```python
from build123d import *

# Parameters (mm, degrees)
CORTE_EXTRUS_O1_DEPTH      = 1
CORTE_EXTRUS_O1_DEPTH_BACK = 51
RESSALTO_EXTRUS_O1_START   = -2
ESBO_O3_R                  = 1.6
RESSALTO_EXTRUS_O1_DEPTH   = 3
ESBO_O4_W                  = 67.372166219
ESBO_O4_H                  = 55.074072385
ESBO_O4_W_2                = 51.598524128
ESBO_O4_H_2                = 14
CORTE_EXTRUS_O2_DEPTH      = 6
CORTE_EXTRUS_O2_DEPTH_BACK = 16.5


with BuildPart() as part:
    # Esboço1 → Revolução1 (revolve)
    with BuildSketch(Plane.XY):
        Polygon((15, 37), (15.5, 37), (15.5, 13), (15, 13), (15, 10), (15.5, 10), (15.5, 0), (12.5, 0), (12.5, 50), (15.5, 50), (15.5, 40), (15, 40), align=None)
    revolve(axis=Axis((0, 0, 0), (0, 1, 0)))

    # Esboço2 → Corte-extrusão1 (cut, two sides)
    with BuildSketch(Plane(origin=(0, 50, 0), x_dir=(1, 0, 0), z_dir=(0, 1, 0))) as corte_extrus_o1_sk:
        with BuildLine():
            Line((-11.456439237, -5), (-14.671400751, -5))
            ThreePointArc((-14.671400751, -5), (0, -15.5), (14.671400751, -5))
            Line((14.671400751, -5), (11.456439237, -5))
            ThreePointArc((11.456439237, -5), (0, -12.5), (-11.456439237, -5))
        make_face()
    extrude(amount=CORTE_EXTRUS_O1_DEPTH, mode=Mode.SUBTRACT)
    extrude(corte_extrus_o1_sk.sketch, amount=-CORTE_EXTRUS_O1_DEPTH_BACK, mode=Mode.SUBTRACT)

    # Esboço3 → Ressalto-extrusão1 (add)
    with BuildSketch(Plane.XY.offset(RESSALTO_EXTRUS_O1_START)):
        with BuildLine():
            Line((-13.5, 49), (-20, 49))
            ThreePointArc((-20, 49), (-24, 45), (-20, 41))
            Line((-20, 41), (-13.5, 41))
            Line((-13.5, 41), (-13.5, 49))
        make_face()
        with Locations((-20, 45)):
            Circle(ESBO_O3_R, mode=Mode.SUBTRACT)
        with BuildLine():
            Line((13.5, 41), (13.5, 49))
            Line((13.5, 49), (20, 49))
            ThreePointArc((20, 49), (24, 45), (20, 41))
            Line((20, 41), (13.5, 41))
        make_face()
        with Locations((20, 45)):
            Circle(ESBO_O3_R, mode=Mode.SUBTRACT)
        with BuildLine():
            Line((13.5, 1), (20, 1))
            ThreePointArc((20, 1), (24, 5), (20, 9))
            Line((20, 9), (13.5, 9))
            Line((13.5, 9), (13.5, 1))
        make_face()
        with Locations((20, 5)):
            Circle(ESBO_O3_R, mode=Mode.SUBTRACT)
        with BuildLine():
            Line((-13.5, 9), (-13.5, 1))
            Line((-13.5, 1), (-20, 1))
            ThreePointArc((-20, 1), (-24, 5), (-20, 9))
            Line((-20, 9), (-13.5, 9))
        make_face()
        with Locations((-20, 5)):
            Circle(ESBO_O3_R, mode=Mode.SUBTRACT)
    extrude(amount=-RESSALTO_EXTRUS_O1_DEPTH)

    # Esboço4 → Corte-extrusão2 (cut, two sides)
    with BuildSketch(Plane.XY) as corte_extrus_o2_sk:
        with Locations((0.066837467, 24.799487601)):
            Rectangle(ESBO_O4_W, ESBO_O4_H)
        with Locations((0, 42)):
            Rectangle(ESBO_O4_W_2, ESBO_O4_H_2, mode=Mode.SUBTRACT)
    extrude(amount=CORTE_EXTRUS_O2_DEPTH, mode=Mode.SUBTRACT)
    extrude(corte_extrus_o2_sk.sketch, amount=-CORTE_EXTRUS_O2_DEPTH_BACK, mode=Mode.SUBTRACT)


solid = part.part
```
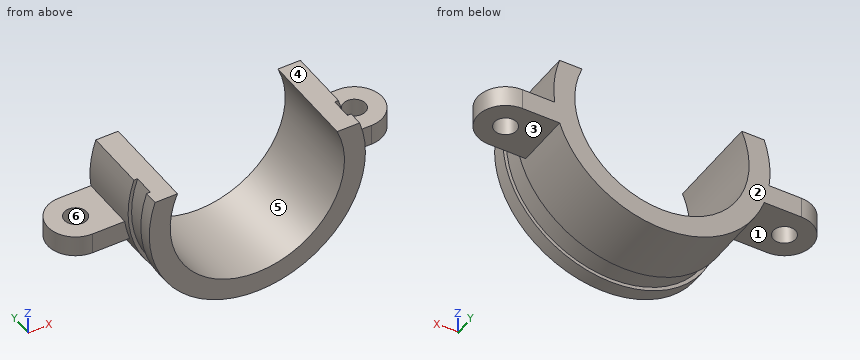
The listing builds one solid part. Answer for the finished solid, in the listing's coordinates (mm). Face numbers are marked on the shaded views. A direction names the side the tool comes from. Give positions to 0.01 mm unless a question says otherwise; leave off trailing zeros. Write each loop counter-clockwise with the first axis right and the second up, starting at its lowest first coordinate (ties: lowest second). Pieces come first, ordered by that corner, then holes. Notation, with made-up numbers: M -19.75,-32 L 18.25,-32 A23 cw 18.25,-8 Z; hole C 44.25,75 d4. An arc over 180 degrees is marked long. Write each question's results on one line, items separated by ' | '.
Q1. Consider L1, parallel to Y at x = -20, z = -4.4; L2, parallel to X at y = 43.75, z = 0; L3, parallel to Y at x = 6, z = -14. Determine where each line is inside the solid, lowest interval first. Write a range as from..to.
Output values:
L1: 41..43.4, 46.6..49 | L2: -15.5..-12.5, 12.5..15.5 | L3: 35..37, 40..49
Q2. Section C-C, the plane x = 0 is taken. Write down the section's boundary in (y, z).
Output values:
outline: M 35,-15.5 L 37,-15.5 L 37,-15 L 40,-15 L 40,-15.5 L 49,-15.5 L 49,-12.5 L 35,-12.5 Z
Q3. A tool of negligible diameter and unlimited length cuts with its end or side. For the marked faces 1 and 2, from which of +Z, -Z, +X, -X, +Y, -Y can it reach the whole face along a straight path? Write none if from no direction.
Output values:
face 1: -Z, -X, +Y, -Y | face 2: +Z, -Z, +X, -X, +Y
Q4. For a pull along Z with two mould halves and no side action, classify the marked faces 3, 4, 5 and 6 as released by +Z, released by -Z, zero draft, split by the parting line, or undercut.
Output values:
face 3: released by -Z | face 4: released by +Z | face 5: undercut | face 6: zero draft
Q5. Section B-B, the plane y = 45 is taken. Write down the section's boundary in (x, z).
Output values:
outline: M -24,-5 L -21.6,-5 L -21.6,-2 L -24,-2 Z; M -18.4,-5 L -14.67,-5 A15.5 ccw 14.67,-5 L 18.4,-5 L 18.4,-2 L 15.37,-2 A15.5 ccw 14.67,5 L 11.46,5 A12.5 cw long -11.46,5 L -14.67,5 A15.5 ccw -15.37,-2 L -18.4,-2 Z; M 21.6,-5 L 24,-5 L 24,-2 L 21.6,-2 Z
Q6. Section A-A, the plane z = -3.25 is taken. Write down the section's boundary in (x, y).
Output values:
outline: M -20,41 L -15.16,41 L -15.16,40 L -14.64,40 L -14.64,37 L -15.16,37 L -15.16,35 L -12.07,35 L -12.07,49 L -20,49 A4 ccw Z; M 12.07,35 L 15.16,35 L 15.16,37 L 14.64,37 L 14.64,40 L 15.16,40 L 15.16,41 L 20,41 A4 ccw 20,49 L 12.07,49 Z; hole C -20,45 d3.2; hole C 20,45 d3.2
Q7. Section D-D, the plane z = 0 is taken. Write down the section's boundary in (x, y).
Output values:
outline: M -15.5,35 L -12.5,35 L -12.5,49 L -15.5,49 L -15.5,40 L -15,40 L -15,37 L -15.5,37 Z; M 12.5,35 L 15.5,35 L 15.5,37 L 15,37 L 15,40 L 15.5,40 L 15.5,49 L 12.5,49 Z
Q8. Flat-ended cylindrical pins translate along their axes: P1, Ø3.5, axis at x = -16, z = -3, coming from the -Y side; P2, Ø5, axis at y = 42.5, z = -12.5, coming from the -X side; P3, Ø6, axis at x = -14.5, y = 37.5, coming from the -Z side; P4, Ø1.5, axis at x = 1, y = 45.5, coming from the +Z side. Find the tip coordinate at first contact, or state that the pin passes through.
Output values:
P1: y = 35 | P2: x = -11.84 | P3: z = -10.35 | P4: z = -12.38
